Verification items for the finished model (mm, model axes). Coordinates: 2 decimals unless noted, no trailing zeros. Write each loop counter-clockwise with the first axis right and the second up, starting at its lowest first coordinate (ties: lowest second). Pieces come first, ordered by that corner, then holes. Notation, with made-up numbers: (26.25, 19.25) -> (30.25, 19.25) arc R30 cw to (30.25, 55.25) -> close; hole circle Ø4 at (-35.5, 77.25). An arc over 180 degrees is marked (long way). Use CSV: the item, a comma, the result in double quotes.
```python
from build123d import *

# Parameters (mm, degrees)
F1_DEPTH = 9.652
F2_W     = 38.7581029464
F2_H     = 3.81
F3_DEPTH = 9.652
F5_DEPTH = 9.652


with BuildPart() as f1:
    # F0 (on Front) → F1 (new body)
    with BuildSketch(Plane.XZ):
        Polygon((0, 9.652), (0, 0), (38.1, 0), (38.1, 2.54), align=None)
    extrude(amount=F1_DEPTH)

    # F2 (on face) → F3 (join)
    with BuildSketch(Plane(origin=(1.7410410582, 0, 9.3270056691), x_dir=(0.9830202488, 0, -0.1834971131), z_dir=(0.1834971131, 0, 0.9830202488))):
        with Locations((17.6079373375, -7.747)):
            Rectangle(F2_W, F2_H)
        with Locations((17.6079373375, -1.905)):
            Rectangle(F2_W, F2_H)
    extrude(amount=F3_DEPTH)

    # F4 (on face) → F5 (join)
    with BuildSketch(Plane.XZ.offset(9.652)):
        Polygon((0, 0), (0, 9.652), (-1.8017066667, 0), align=None)
    extrude(amount=-F5_DEPTH)


solid = f1.part
```
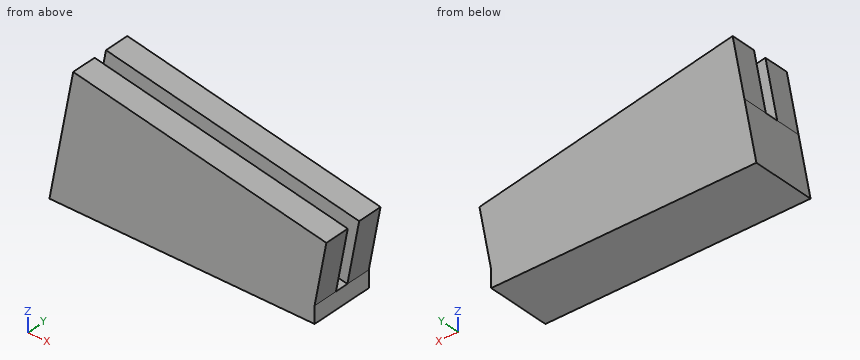
1) Cross-section at A-A (z = 11.5). Record the boundary of the cut face in (x, y).
Return value:
outline,"(0.34, -9.65) -> (39.77, -9.65) -> (39.77, -5.84) -> (0.34, -5.84) -> close; (0.34, -3.81) -> (39.77, -3.81) -> (39.77, 0) -> (0.34, 0) -> close"
2) Scan lines: L1, parallel to Y at x = 5, z = 14.75; L2, parallel to Z at x = 26.5, y = -6; L3, parallel to X at y = -3.5, z = 8. Record each from-to range of solid material in increasing order.
Return value:
L1,"-9.65 to -5.84, -3.81 to 0"
L2,"0 to 14.52"
L3,"-0.31 to 39.12"
3) Cross-section at C-C (x = 22). Record the boundary of the cut face in (y, z), plus the area to 3 significant figures.
Return value:
outline,"(-9.65, 0) -> (0, 0) -> (0, 15.36) -> (-3.81, 15.36) -> (-3.81, 5.55) -> (-5.84, 5.55) -> (-5.84, 15.36) -> (-9.65, 15.36) -> close"
area,"128 mm2"
4) Cross-section at D-D (z = 15). Record the boundary of the cut face in (x, y).
Return value:
outline,"(1, -9.65) -> (23.95, -9.65) -> (23.95, -5.84) -> (1, -5.84) -> close; (1, -3.81) -> (23.95, -3.81) -> (23.95, 0) -> (1, 0) -> close"
5) Cross-section at B-B (y = -8.25). Record the boundary of the cut face in (x, z).
Return value:
outline,"(-1.8, 0) -> (38.1, 0) -> (38.1, 2.54) -> (39.87, 12.03) -> (1.77, 19.14) -> close"
6) Gauge pin test, flat ends, axial feed: pin 1 (4 mm diameter, centred on y = -7.5, z = 2.5, fed in from +X); pin 2 (0.8 mm diameter, centred on y = -3, z = 1, fed in from +X). Record the tip position at first contact, or that the pin passes through.
Return value:
pin 1,"x = 38.47"
pin 2,"x = 38.1"
